Check sheet for the modelled part. Datum: model origin and axes. Units: mm. A direction names the side the tool comes from. Round coordinates to 2 decimals unless told otherwise and drop trailing zeros. Write each loop counter-clockwise with the first axis right and the second up, starting at its lowest first coordinate (ties: lowest second). Pieces come first, ordered by that corner, then holes. Notation, with made-up numbers: (83.5, 4) -> (91.5, 4) arc R14 ccw to (91.5, 11) -> close; hole circle Ø8 at (10.5, 39). An arc over 180 degrees is marked (long way). Write item = value, one per line.
from build123d import *

# Parameters (mm, degrees)
BOSS_EXTRUDE1_DEPTH = 2
SKETCH3_W           = 2.15
SKETCH3_H           = 30
SKETCH4_W           = 2.15
SKETCH4_H           = 30
SKETCH6_R           = 1.5
CUT_EXTRUDE1_DEPTH  = 29


with BuildPart() as part:
    # Sketch2 → Boss-Extrude1 (new body)
    with BuildSketch(Plane.XY):
        with BuildLine():
            Line((-20.5, -1), (-13.5, -1))
            ThreePointArc((-13.5, -1), (-12.085786438, -0.414213562), (-11.5, 1))
            Line((-11.5, 1), (-11.5, 7))
            ThreePointArc((-11.5, 7), (-11, 7.5), (-10.5, 7))
            Line((-10.5, 7), (-10.5, 0))
            Line((-10.5, 0), (-10.5, -7))
            ThreePointArc((-10.5, -7), (-8, -9.5), (-5.5, -7))
            Line((-5.5, -7), (-5.5, 0))
            Line((-5.5, 0), (-5.5, 7))
            ThreePointArc((-5.5, 7), (-5, 7.5), (-4.5, 7))
            Line((-4.5, 7), (-4.5, 0))
            Line((-4.5, 0), (-4.5, -7))
            ThreePointArc((-4.5, -7), (-2, -9.5), (0.5, -7))
            Line((0.5, -7), (0.5, 0))
            Line((0.5, 0), (0.5, 7))
            ThreePointArc((0.5, 7), (1, 7.5), (1.5, 7))
            Line((1.5, 7), (1.5, 0))
            Line((1.5, 0), (1.5, -7))
            ThreePointArc((1.5, -7), (4, -9.5), (6.5, -7))
            Line((6.5, -7), (6.5, -1))
            Line((6.5, -1), (13.5, -1))
            ThreePointArc((13.5, -1), (14.5, 0), (13.5, 1))
            Line((13.5, 1), (6.5, 1))
            ThreePointArc((6.5, 1), (5.085786438, 0.414213562), (4.5, -1))
            Line((4.5, -1), (4.5, -7))
            ThreePointArc((4.5, -7), (4, -7.5), (3.5, -7))
            Line((3.5, -7), (3.5, 0))
            Line((3.5, 0), (3.5, 7))
            ThreePointArc((3.5, 7), (1, 9.5), (-1.5, 7))
            Line((-1.5, 7), (-1.5, 0))
            Line((-1.5, 0), (-1.5, -7))
            ThreePointArc((-1.5, -7), (-2, -7.5), (-2.5, -7))
            Line((-2.5, -7), (-2.5, 0))
            Line((-2.5, 0), (-2.5, 7))
            ThreePointArc((-2.5, 7), (-5, 9.5), (-7.5, 7))
            Line((-7.5, 7), (-7.5, 0))
            Line((-7.5, 0), (-7.5, -7))
            ThreePointArc((-7.5, -7), (-8, -7.5), (-8.5, -7))
            Line((-8.5, -7), (-8.5, 0))
            Line((-8.5, 0), (-8.5, 7))
            ThreePointArc((-8.5, 7), (-11, 9.5), (-13.5, 7))
            Line((-13.5, 7), (-13.5, 1))
            Line((-13.5, 1), (-20.5, 1))
            ThreePointArc((-20.5, 1), (-21.5, 0), (-20.5, -1))
        make_face()
    extrude(amount=BOSS_EXTRUDE1_DEPTH)

    # Sketch3 → Revolve1 (revolve)
    with BuildSketch(Plane(origin=(0, 0, 0), x_dir=(1, 0, 0), z_dir=(0, 1, 0)), mode=Mode.PRIVATE) as revolve1_sk:
        with Locations((-21.575, 13)):
            Rectangle(SKETCH3_W, SKETCH3_H)
    revolve(revolve1_sk.sketch.rotate(Axis((-20.5, 0, 2), (0, 0, -1)), 180), axis=Axis((-20.5, 0, 2), (0, 0, -1)))

    # Sketch4 → Revolve2 (revolve)
    with BuildSketch(Plane(origin=(0, 0, 0), x_dir=(1, 0, 0), z_dir=(0, 1, 0))):
        with Locations((14.575, 13)):
            Rectangle(SKETCH4_W, SKETCH4_H)
    revolve(axis=Axis((13.5, 0, 2), (0, 0, -1)))

    # Sketch6 → Cut-Extrude1 (cut)
    with BuildSketch(Plane(origin=(0, 0, -28), x_dir=(-1, 0, 0), z_dir=(0, 0, -1))):
        with Locations((-13.5, 0)):
            Circle(SKETCH6_R)
        with Locations((20.5, 0)):
            Circle(SKETCH6_R)
    extrude(amount=-CUT_EXTRUDE1_DEPTH, mode=Mode.SUBTRACT)


solid = part.part
(1) Sectioned sample at B-B on y = 6. Enter the section's corners in (x, z).
Worked answers:
outline = (-13.5, 0) -> (-11.5, 0) -> (-11.5, 2) -> (-13.5, 2) -> close; (-10.5, 0) -> (-8.5, 0) -> (-8.5, 2) -> (-10.5, 2) -> close; (-7.5, 0) -> (-5.5, 0) -> (-5.5, 2) -> (-7.5, 2) -> close; (-4.5, 0) -> (-2.5, 0) -> (-2.5, 2) -> (-4.5, 2) -> close; (-1.5, 0) -> (0.5, 0) -> (0.5, 2) -> (-1.5, 2) -> close; (1.5, 0) -> (3.5, 0) -> (3.5, 2) -> (1.5, 2) -> close
(2) Release check for a two-part mould opening along Y. For faces 1 (the cylindrical face through (3.9, -9.5, 1)), 2 (the flat face through (14, 0, 1)), 3 (the cylindrical face through (15, 0, -14)), 4 (the flat face through (-3, 0, 2)) record: pulls with the +Y half, pulls with the -Y half, needs draft (parallel to the pull), parting line crosses it, or undercut.
Worked answers:
face_1 = pulls with the -Y half
face_2 = undercut
face_3 = undercut
face_4 = needs draft
(3) Access from +Z, -Z, +X, -X, +Y, -Y to the whole of each face (thin tool, end or side, straight path). Record for faces 5 (the flat face through (-20, 0, 1)), 6 (the flat face through (-7.5, 0, 1)), 7 (the flat face through (-4.5, 0, 1)).
Worked answers:
face_5 = -Z
face_6 = +Z, -Z, +Y
face_7 = +Z, -Z, -Y
(4) Sectioned sample at D-D on y = 0. Count the separate pieces of the cut face and the enclosed holes in it, then the cut area to 3 significant figures.
Worked answers:
separate_pieces = 7
enclosed_holes = 0
area = 130 mm²
(5) Sectioned sample at A-A on z = -11. Enter the section's corners in (x, y), then the cut area to 3 significant figures.
Worked answers:
outline = circle Ø4.3 at (-20.5, 0); circle Ø4.3 at (13.5, 0); hole circle Ø3 at (-20.5, 0); hole circle Ø3 at (13.5, 0)
area = 14.9 mm²
(6) Sectioned sample at C-C on x = -9.5. Enter the section's corners in (y, z).
Worked answers:
outline = (-9, 0) -> (9, 0) -> (9, 2) -> (-9, 2) -> close
(7) Material ranges on L1, parallel to Y at x = -20.5, z = -21; L2, parallel to Z at x = 3, y = -0.5; L3, parallel to Z at x = 13, y = -1.25, recorded low to high. Write a range as [from, to].
Worked answers:
L1 = [-2.15, -1.5], [1.5, 2.15]
L2 = [0, 2]
L3 = [1, 2]
(8) Go/stop test with flat-tipped pins: P1, Ø0.6, axis at y = 3, z = 1, coming from the +X side; P2, Ø1, axis at y = 1, z = 0.5, coming from the -X side; P3, Ø1, axis at x = 9, z = 0.5, coming from the +Y side; P4, Ø2.5, axis at x = -21, y = 0, coming from the -Z side. Record where each tip stops, or that it passes through.
Worked answers:
P1 = 3.5
P2 = -22.59
P3 = 1
P4 = -28
